from build123d import *

# Parameters (mm, degrees)
ESBO_O1_W                      = 660
ESBO_O1_H                      = 230
RESSALTO_EXTRUS_O1_DEPTH       = 32
FILETE1_RADIUS                 = 16
FILETE1_LENGTH                 = 230
FILETE2_RADIUS                 = 16
FILETE2_LENGTH                 = 230
ESBO_O2_R                      = 5
RESSALTO_EXTRUS_O2_DEPTH       = 10
PADR_O_LINEAR1_COUNT           = 3
PADR_O_LINEAR1_PITCH           = 150
PADR_O_LINEAR1_COPY_1_SKETCH_R = 5
PADR_O_LINEAR1_COPY_1_DEPTH    = 10
PADR_O_LINEAR1_COPY_2_SKETCH_R = 5
PADR_O_LINEAR1_COPY_2_DEPTH    = 10
ESBO_O6_R                      = 5
RESSALTO_EXTRUS_O7_DEPTH       = 5
ESBO_O10_W                     = 20
ESBO_O10_H                     = 5
RESSALTO_EXTRUS_O11_DEPTH      = 5
PADR_O_LINEAR2_COUNT           = 3
PADR_O_LINEAR2_PITCH           = 150
RESSALTO_EXTRUS_O10_DEPTH      = 5
ESPELHAR2_COPY_1_SKETCH_R      = 5
ESPELHAR2_COPY_1_DEPTH         = 5
ESPELHAR2_COPY_2_SKETCH_R      = 5
ESPELHAR2_COPY_2_DEPTH         = 5
ESPELHAR2_COPY_3_SKETCH_W      = 20
ESPELHAR2_COPY_3_SKETCH_H      = 5
ESPELHAR2_COPY_3_DEPTH         = 5
ESPELHAR2_COPY_4_SKETCH_W      = 20
ESPELHAR2_COPY_4_SKETCH_H      = 5
ESPELHAR2_COPY_4_DEPTH         = 5


with BuildPart() as part:
    # Esboço1 → Ressalto-extrusão1 (new body)
    with BuildSketch(Plane(origin=(0, 0, 0), x_dir=(1, 0, 0), z_dir=(0, 1, 0))):
        with Locations((330, 115)):
            Rectangle(ESBO_O1_W, ESBO_O1_H)
    extrude(amount=RESSALTO_EXTRUS_O1_DEPTH)

    # Filete1: full round fillet: the end face becomes a half cylinder, R = half its width
    filete1_face = Plane((0, 16, -115), x_dir=(0, 0, -1), z_dir=(-1, 0, 0))  # on the end face: x along it, z out of the body
    filete1_slab = filete1_face.offset(-FILETE1_RADIUS / 2) * Box(FILETE1_LENGTH, 2 * FILETE1_RADIUS, FILETE1_RADIUS, mode=Mode.PRIVATE)  # the body's end, R deep
    filete1_round = Plane((16, 16, -115), x_dir=(-1, 0, 0), z_dir=(0, 0, -1)) * Cylinder(FILETE1_RADIUS, FILETE1_LENGTH, mode=Mode.PRIVATE)  # its axis R under the face
    add(filete1_slab - filete1_round, mode=Mode.SUBTRACT)

    # Filete2: full round fillet: the end face becomes a half cylinder, R = half its width
    filete2_face = Plane((660, 16, -115), x_dir=(0, 0, 1), z_dir=(1, 0, 0))  # on the end face: x along it, z out of the body
    filete2_slab = filete2_face.offset(-FILETE2_RADIUS / 2) * Box(FILETE2_LENGTH, 2 * FILETE2_RADIUS, FILETE2_RADIUS, mode=Mode.PRIVATE)  # the body's end, R deep
    filete2_round = Plane((644, 16, -115), x_dir=(1, 0, 0), z_dir=(0, 0, 1)) * Cylinder(FILETE2_RADIUS, FILETE2_LENGTH, mode=Mode.PRIVATE)  # its axis R under the face
    add(filete2_slab - filete2_round, mode=Mode.SUBTRACT)

    # Esboço2 → Ressalto-extrusão2 (add)
    with BuildSketch(Plane.XY):
        with Locations(Location((150.5, 16, 0), (0, 0, 180))):
            Circle(ESBO_O2_R)
    ressalto_extrus_o2 = extrude(amount=RESSALTO_EXTRUS_O2_DEPTH)

    # Espelhar1: Ressalto-extrusão2 across plane
    add(ressalto_extrus_o2.mirror(Plane.XY.offset(-115)))

    # Padrão linear1: Ressalto-extrusão2 ×3
    with Locations(*[(i * PADR_O_LINEAR1_PITCH, 0, 0) for i in range(1, PADR_O_LINEAR1_COUNT)]):
        add(ressalto_extrus_o2)

    # Padrão linear1 copy 1 sketch → Padrão linear1 copy 1 (add)
    with BuildSketch(Plane(origin=(150, 0, -230), x_dir=(1, 0, 0), z_dir=(0, 0, -1))):
        with Locations((150.5, -16)):
            Circle(PADR_O_LINEAR1_COPY_1_SKETCH_R)
    extrude(amount=PADR_O_LINEAR1_COPY_1_DEPTH)

    # Padrão linear1 copy 2 sketch → Padrão linear1 copy 2 (add)
    with BuildSketch(Plane(origin=(300, 0, -230), x_dir=(1, 0, 0), z_dir=(0, 0, -1))):
        with Locations((150.5, -16)):
            Circle(PADR_O_LINEAR1_COPY_2_SKETCH_R)
    extrude(amount=PADR_O_LINEAR1_COPY_2_DEPTH)

    # Esboço6 → Ressalto-extrusão7 (add)
    with BuildSketch(Plane.XY):
        with BuildLine():
            Line((140.5, 16), (140.5, 46))
            Line((140.5, 46), (160.5, 46))
            Line((160.5, 46), (160.5, 16))
            ThreePointArc((160.5, 16), (150.5, 6), (140.5, 16))
        make_face()
        with Locations((150.5, 16)):
            Circle(ESBO_O6_R, mode=Mode.SUBTRACT)
    ressalto_extrus_o7 = extrude(amount=RESSALTO_EXTRUS_O7_DEPTH)

    # Esboço10 → Ressalto-extrusão11 (add)
    with BuildSketch(Plane(origin=(0, 0, 0), x_dir=(-1, 0, 0), z_dir=(0, 0, -1))):
        with Locations((-150.5, 35.5)):
            Rectangle(ESBO_O10_W, ESBO_O10_H)
    ressalto_extrus_o11 = extrude(amount=RESSALTO_EXTRUS_O11_DEPTH)

    # Padrão linear2: Ressalto-extrusão7, Ressalto-extrusão11 ×3
    with Locations(*[(i * PADR_O_LINEAR2_PITCH, 0, 0) for i in range(1, PADR_O_LINEAR2_COUNT)]):
        add(ressalto_extrus_o7)
        add(ressalto_extrus_o11)

    # Esboço9 → Ressalto-extrusão10 (add)
    with BuildSketch(Plane(origin=(0, 46, 0), x_dir=(1, 0, 0), z_dir=(0, 1, 0))):
        Polygon((160.5, -5), (160.5, 10), (290.5, 10), (290.5, -5), (310.5, -5), (310.5, 10), (440.5, 10), (440.5, -5), (460.5, -5), (460.5, 55), (110.5, 80), (140.5, 10), (140.5, -5), align=None)
    ressalto_extrus_o10 = extrude(amount=RESSALTO_EXTRUS_O10_DEPTH)

    # Espelhar2: Ressalto-extrusão7, Ressalto-extrusão11, Ressalto-extrusão10 across plane
    add(ressalto_extrus_o7.mirror(Plane(origin=(0, 0, -115), x_dir=(1, 0, 0), z_dir=(0, 0, -1))))
    add(ressalto_extrus_o11.mirror(Plane(origin=(0, 0, -115), x_dir=(1, 0, 0), z_dir=(0, 0, -1))))
    add(ressalto_extrus_o10.mirror(Plane(origin=(0, 0, -115), x_dir=(1, 0, 0), z_dir=(0, 0, -1))))

    # Espelhar2 copy 1 sketch → Espelhar2 copy 1 (add)
    with BuildSketch(Plane(origin=(150, 0, -230), x_dir=(1, 0, 0), z_dir=(0, 0, -1))):
        with BuildLine():
            Line((140.5, -16), (140.5, -46))
            Line((140.5, -46), (160.5, -46))
            Line((160.5, -46), (160.5, -16))
            ThreePointArc((160.5, -16), (150.5, -6), (140.5, -16))
        make_face()
        with Locations((150.5, -16)):
            Circle(ESPELHAR2_COPY_1_SKETCH_R, mode=Mode.SUBTRACT)
    extrude(amount=ESPELHAR2_COPY_1_DEPTH)

    # Espelhar2 copy 2 sketch → Espelhar2 copy 2 (add)
    with BuildSketch(Plane(origin=(300, 0, -230), x_dir=(1, 0, 0), z_dir=(0, 0, -1))):
        with BuildLine():
            Line((140.5, -16), (140.5, -46))
            Line((140.5, -46), (160.5, -46))
            Line((160.5, -46), (160.5, -16))
            ThreePointArc((160.5, -16), (150.5, -6), (140.5, -16))
        make_face()
        with Locations((150.5, -16)):
            Circle(ESPELHAR2_COPY_2_SKETCH_R, mode=Mode.SUBTRACT)
    extrude(amount=ESPELHAR2_COPY_2_DEPTH)

    # Espelhar2 copy 3 sketch → Espelhar2 copy 3 (add)
    with BuildSketch(Plane(origin=(150, 0, -230), x_dir=(-1, 0, 0), z_dir=(0, 0, 1))):
        with Locations((-150.5, -35.5)):
            Rectangle(ESPELHAR2_COPY_3_SKETCH_W, ESPELHAR2_COPY_3_SKETCH_H)
    extrude(amount=ESPELHAR2_COPY_3_DEPTH)

    # Espelhar2 copy 4 sketch → Espelhar2 copy 4 (add)
    with BuildSketch(Plane(origin=(300, 0, -230), x_dir=(-1, 0, 0), z_dir=(0, 0, 1))):
        with Locations((-150.5, -35.5)):
            Rectangle(ESPELHAR2_COPY_4_SKETCH_W, ESPELHAR2_COPY_4_SKETCH_H)
    extrude(amount=ESPELHAR2_COPY_4_DEPTH)


solid = part.part
Build history of the part. All positions in model axes, mm. A direction names the side the tool comes from. Give positions to 0.01 mm unless a question says otherwise; leave off trailing zeros. Order: outer loops, then holes, each group sorted by start corner. A loop starts at its lowest first (then second) coordinate and runs counter-clockwise, first axis right, second up. Notation, with made-up numbers: M -29.75,66.5 L 26.25,66.5 A18 ccw 26.25,80.5 Z; hole C 50,0 d7. An arc over 180 degrees is marked long. Use one line per item in the form item = value.
1) Two-plate mould, pull along X, no slides. Class faces 5 (the face through (310.5, 38, -231)), 6 (the face through (140.5, 37, -231)), 7 (the face through (283, 46, -189)): released by +X, released by -X, zero draft, split by the parting line, or undercut.
Calculated:
face_5 = undercut
face_6 = released by -X
face_7 = zero draft
2) Drop flat-ended pins along their axis: pin 1 (3 mm diameter, centred on x = 265.5, y = 20.5, fed in from +Z); pin 2 (1.5 mm diameter, centred on x = 521, z = -201.5, fed in from +Y); pin 3 (4 mm diameter, centred on x = 491.5, z = -188, fed in from -Y); pin 4 (6 mm diameter, centred on x = 149, y = 35.5, fed in from -Z). Give the stop position or say it passes through.
Calculated:
pin_1 = 0
pin_2 = 32
pin_3 = 0
pin_4 = -235
3) Saw through at C-C (z = -93.5). Give the cut face in (x, y), plus the area to 3 significant figures.
Calculated:
outline = M 16,0 L 644,0 A16 ccw 644,32 L 16,32 A16 ccw Z
area = 20,900 mm2
4) Tool access for faces 1 (the face through (310.5, 37, 1)), 2 (the face through (140.5, 37, 1)), 3 (the face through (290.5, 37, -231)), 4 (the face through (287.95, 48.465, -67.325)): list every direction of +Z, -Z, +X, -X, +Y, -Y with a clear straight run to the whole face (end or side of a thin tool).
Calculated:
face_1 = +Z, +Y
face_2 = +Z, -X, +Y
face_3 = -Z, +Y
face_4 = +X, +Y
5) Probe probe 1 along Y at (x, z) = (445, -201.5); probe 2 along Z at (x, y) = (158, 42); probe 3 along Y at (x, z) = (167.5, -111.5). List the from-to ranges inside material, lowest first.
Calculated:
probe_1 = 0 to 32, 46 to 51
probe_2 = -235 to -230, 0 to 5
probe_3 = 0 to 32
6) Saw through at B-B (z = -45.5). Give the cut face in (x, y), plus the area to 3 significant figures.
Calculated:
outline = M 16,0 L 644,0 A16 ccw 644,32 L 16,32 A16 ccw Z; M 125.29,46 L 460.5,46 L 460.5,51 L 125.29,51 Z
area = 22,600 mm2
7) Saw through at D-D (x = 102). Give the cut face in (y, z), plus the area to 3 significant figures.
Calculated:
outline = M 0,-230 L 32,-230 L 32,0 L 0,0 Z
area = 7,360 mm2
8) Saw through at A-A (x = 407.5). Give the cut face in (y, z).
Calculated:
outline = M 0,-230 L 32,-230 L 32,0 L 0,0 Z; M 46,-220 L 51,-220 L 51,-171.21 L 46,-171.21 Z; M 46,-58.79 L 51,-58.79 L 51,-10 L 46,-10 Z
